Geometry check sheet. Reference: the model listing, model coordinates, mm. A direction names the side the tool comes from. Round coordinates to 2 decimals unless told otherwise and drop trailing zeros. Order: outer loops, then holes, each group sorted by start corner. A loop starts at its lowest first (then second) coordinate and runs counter-clockwise, first axis right, second up. Notation, with made-up numbers: (24.5, -34.75) - (47.5, -34.75) arc R19 cw to (47.5, 1.25) - close; hole circle Ø3 at (-13, 72). An arc over 180 degrees is marked (long way). Return JSON: item names as keys, results as strings. Group by question number.
Q1. Material ranges on line 1 along Y through (x, z) = (-2, 0); line 2 along Y through (x, z) = (12, 0), recorded low to high.
Q2. Sectioned sample at C-C, the plane x = 18. Record the cut outline in (y, z).
Q3. Sectioned sample at A-A, the plane y = 0. Record the cut outline in (x, z), then the cut area to 3 significant figures.
Q4. Tool access check on faces 4 (the conical face through (-14.156, -11.09, 5.768)), 5 (the cylindrical face through (19.72, -7.81, -1.73)), 6 (the cylindrical face through (-1.774, -19.524, -4.336)). Record the directions out of +Z, -Z, +X, -X, +Y, -Y that give a thin tool (end or side, any length) a straight path to the whole face; none if there is none.
Q5. Gauge pin test, flat ends, axial feed: pin 1 Ø1 at (x, z) = (20.5, -1) entering from +Y; pin 2 Ø6 at (y, z) = (12.5, -9) entering from +X; pin 3 Ø10 at (x, z) = (-13, -4) entering from -Y. Record the tip position at first contact, or that the pin passes through.
Q6. Sectioned sample at D-D, the plane x = -5. Record the cut outline in (y, z), then the cut area to 3 significant figures.
Q7. Draft check along Z on faces 1 (the conical face through (-5.844, 11.09, 5.768)), 2 (the cylindrical face through (9.58, -4.88, -1.08)), 3 (the flat face through (-20, 4, 4)). Enter one of: pulls with the +Z half, pulls with the -Z half, needs draft (parallel to the pull), parting line crosses it, or undercut.
Autodesk Inventor part; units mm, degrees
ref_plane "YZ Plane" through (0, 0, 0) normal (1, 0, 0) x (0, 1, 0)
ref_plane "XZ Plane" through (0, 0, 0) normal (0, 1, 0) x (-1, 0, 0)
ref_plane "XY Plane" through (0, 0, 0) normal (0, 0, 1) x (1, 0, 0)
sketch "Эскиз1" plane through (0, 0, 0) normal (0, 1, 0) x (-1, 0, 0)
  line L0 (0, 20) -> (20, 20)
  line L1 (20, 20) -> (20, 0)
  line L2 (20, 0) -> (0, 0)
  line L3 (20, 20) -> (14, 20)
  line L4 (14, 20) -> (14, 12)
  line L5 (14, 12) -> (6, 12)
  line L6 (6, 12) -> (6, 20)
  line L7 (20, 0) -> (-40, 0)
  line L8 (-40, 0) -> (-40, 8)
  line L9 (-40, 8) -> (0, 8)
  line L10 (-40, 0) -> (-40, 5)
  line L11 (-40, 5) -> (20, 5)
  line L12 (0, 0) -> (0, 5)
  line L13 (0, 8) -> (0, 20)
  line L14 (10, 12) -> (10, 20)
  line L15 (10, 20) -> (3.5, 20)
  line L16 (3.5, 20) -> (6, 12)
  line L17 (3.5, 20) -> (16.5, 20)
  line L18 (16.5, 20) -> (14, 12)
  dimension "d0" = 20
  dimension "d1" = 20
  dimension "d2" = 6
  dimension "d3" = 8
  dimension "d4" = 8
  dimension "d5" = 60
  dimension "d6" = 8
  dimension "d7" = 5
  dimension "d15" = 6.5
  dimension "d16" = 13
revolve "Вращение1" add sketch "Эскиз1" angle 360 about axis through (-20, 0, 0) along (1, 0, 0) contours L0 L16 L5 L18 L1 L11 L8 L9 L13
properties part number "Шкив 20"
Reply:
{
 "1": {"line 1": "-20 to -5, 5 to 20", "line 2": "-8 to -5, 5 to 8"},
 "2": {"outline": "circle Ø16 at (0, 0); hole circle Ø10 at (0, 0)"},
 "3": {"outline": "(-20, -20) - (-16.5, -20) - (-14, -12) - (-6, -12) - (-3.5, -20) - (0, -20) - (0, -8) - (40, -8) - (40, -5) - (-20, -5) - close; (-20, 5) - (40, 5) - (40, 8) - (0, 8) - (0, 20) - (-3.5, 20) - (-6, 12) - (-14, 12) - (-16.5, 20) - (-20, 20) - close", "area": "672 mm^2"},
 "4": {"face 4": "none", "face 5": "+X", "face 6": "+X, -X"},
 "5": {"pin 1": "y = 7.98", "pin 2": "x = 0", "pin 3": "y = -20"},
 "6": {"outline": "circle Ø30.4 at (0, 0); hole circle Ø10 at (0, 0)", "area": "647 mm^2"},
 "7": {"face 1": "parting line crosses it", "face 2": "undercut", "face 3": "needs draft"}
}
